Build history of the part. All positions in model axes, mm. Face numbers are marked on the shaded views. A direction names the side the tool comes from. Round coordinates to 2 decimals unless told otherwise and drop trailing zeros. Order: outer loops, then holes, each group sorted by start corner. A loop starts at its lowest first (then second) coordinate and runs counter-clockwise, first axis right, second up. Notation, with made-up numbers: (3, 73.5) -> (53, 73.5) arc R34 ccw to (53, 106.5) -> close; hole circle Ø1 at (59, -22.5). An arc over 180 degrees is marked (long way). Use a Markdown table: item, result. Add a question column.
Item 1: Slice it at B-B, the plane x = 0. Give the cut face in (y, z).
Item 2: Slice it at C-C, the plane y = -3. Give the cut face in (x, z).
Item 3: Slice it at A-A, the plane y = 2.5. Give the cut face in (x, z).
Item 4: Two-plate mould, pull along X, no slides. Class the marked faces 1, 2 and 3: released by +X, released by -X, zero draft, split by the parting line, or undercut.
Item 5: Probe L1, parallel to Y at x = -1, z = -0.25; L2, parallel to Y at x = 1.25, z = 3; L3, parallel to Z at x = -1, y = 1. List the from-to ranges inside material, lowest first.
Item 6: 3-axis set-ups, long thin cutter, end or side, ignore diameter. For the marked faces 4, 5 and 6: which of +Z, -Z, +X, -X, +Y, -Y reach the whole face in a straight line?
Item 7: Pin check, flat tip, straight feed: pin 1 (1 mm diameter, centred on y = -3.5, z = 1, fed in from +X). Stop position of the tip, or through.
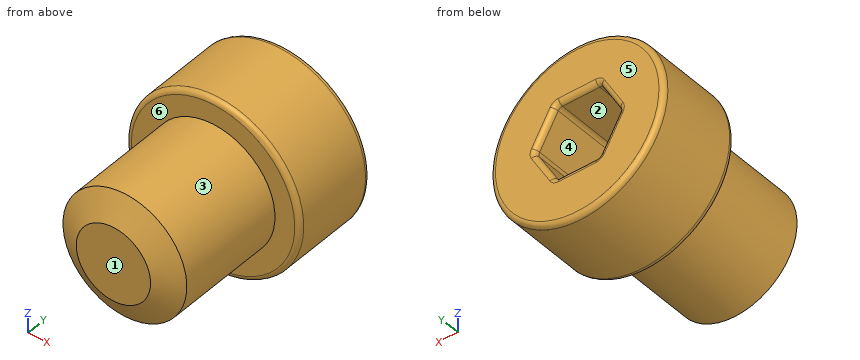
from build123d import *

# Parameters (mm, degrees)
HEAD_SKETCH_R                  = 3.5
HEAD_DEPTH                     = 3.5
THREADED_SECTION_STUB_SKETCH_R = 2.5
THREADED_SECTION_DEPTH         = 5
COSMETIC_FILLETS_R             = 0.2
BOTTOM_CHAMFER_SIZE            = 1
BOTTOM_CHAMFER_SIZE2           = 0.577350269


with BuildPart() as part:
    # Head Sketch → Head (new body)
    with BuildSketch(Plane(origin=(0, 0, 0), x_dir=(1, 0, 0), z_dir=(0, 1, 0))):
        with Locations(Location((0, 0, 0), (0, 0, 270))):
            Circle(HEAD_SKETCH_R)
        Polygon((-0.866025404, 1.5), (-1.732050808, 0), (-0.866025404, -1.5), (0.866025404, -1.5), (1.732050808, 0), (0.866025404, 1.5), align=None, mode=Mode.SUBTRACT)
    extrude(amount=HEAD_DEPTH)

    # Threaded Section Stub Sketch → Threaded Section (add)
    with BuildSketch(Plane(origin=(0, 0, 0), x_dir=(1, 0, 0), z_dir=(0, 1, 0))):
        with Locations(Location((0, 0, 0), (0, 0, 270))):
            Circle(THREADED_SECTION_STUB_SKETCH_R)
    extrude(amount=-THREADED_SECTION_DEPTH)

    # Cosmetic Fillets
    cosmetic_fillets_edges = [part.edges().sort_by_distance(p)[0] for p in [
        (-0.866025404, 1.75, -1.5),
        (-1.299038106, 0, 0.75),
        (-1.732050808, 1.75, 0),
        (0, 0, 1.5),
        (-0.866025404, 1.75, 1.5),
        (1.299038106, 0, 0.75),
        (0.866025404, 1.75, 1.5),
        (1.299038106, 0, -0.75),
        (1.732050808, 1.75, 0),
        (0, 3.5, -1.5),
        (-1.299038106, 3.5, -0.75),
        (-1.299038106, 3.5, 0.75),
        (0, 3.5, 1.5),
        (1.299038106, 3.5, 0.75),
        (1.299038106, 3.5, -0.75),
        (0, 0, -3.5),
        (0, 3.5, -3.5),
        (0, 0, -1.5),
        (0.866025404, 1.75, -1.5),
        (-1.299038106, 0, -0.75),
    ]]
    fillet(cosmetic_fillets_edges, radius=COSMETIC_FILLETS_R)

    # Bottom Chamfer
    bottom_chamfer_edges = [part.edges().sort_by_distance(p)[0] for p in [
        (0, -5, -2.5),
    ]]
    bottom_chamfer_side = [part.faces().sort_by_distance(p)[0] for p in [
        (0, -5, 0),
    ]]
    chamfer(bottom_chamfer_edges, length=BOTTOM_CHAMFER_SIZE, length2=BOTTOM_CHAMFER_SIZE2, reference=bottom_chamfer_side[0])


solid = part.part
Check sheet entries:
| question | item | result |
|---|---|---|
| 1 | outline | (-5, -1.5) -> (-4.42, -2.5) -> (0, -2.5) -> (0, -3.3) arc R0.2 ccw to (0.2, -3.5) -> (3.3, -3.5) arc R0.2 ccw to (3.5, -3.3) -> (3.5, -1.7) arc R0.2 ccw to (3.3, -1.5) -> (0.2, -1.5) arc R0.2 cw to (0, -1.3) -> (0, 1.3) arc R0.2 cw to (0.2, 1.5) -> (3.3, 1.5) arc R0.2 ccw to (3.5, 1.7) -> (3.5, 3.3) arc R0.2 ccw to (3.3, 3.5) -> (0.2, 3.5) arc R0.2 ccw to (0, 3.3) -> (0, 2.5) -> (-4.42, 2.5) -> (-5, 1.5) -> close |
| 2 | outline | circle Ø5 at (0, 0) |
| 3 | outline | circle Ø7 at (0, 0); hole (-1.67, -0.1) -> (-0.92, -1.4) arc R0.2 ccw to (-0.75, -1.5) -> (0.75, -1.5) arc R0.2 ccw to (0.92, -1.4) -> (1.67, -0.1) arc R0.2 ccw to (1.67, 0.1) -> (0.92, 1.4) arc R0.2 ccw to (0.75, 1.5) -> (-0.75, 1.5) arc R0.2 ccw to (-0.92, 1.4) -> (-1.67, 0.1) arc R0.2 ccw to start |
| 4 | face 1 | zero draft |
| 4 | face 2 | undercut |
| 4 | face 3 | split by the parting line |
| 5 | L1 | -5 to 0 |
| 5 | L2 | 0 to 3.5 |
| 5 | L3 | -3.35 to -1.27, 1.27 to 3.35 |
| 6 | face 4 | +Y |
| 6 | face 5 | +Z, -Z, +X, -X, +Y |
| 6 | face 6 | -Y |
| 7 | pin 1 | x = 2.45 |
